```python
from build123d import *

# Parameters (mm, degrees)
F0_W     = 41.5
F0_H     = 36.8
F1_DEPTH = 20
F2_W     = 55
F2_H     = 2.5
F3_DEPTH = 20
F4_R     = 3
F5_DEPTH = 5
F6_R     = 2.25
F7_DEPTH = 25
F8_R     = 2


with BuildPart() as f1:
    # F0 (on Front) → F1 (new body)
    with BuildSketch(Plane.XZ):
        Rectangle(F0_W, F0_H)
    extrude(amount=F1_DEPTH)

    # F2 (on face) → F3 (join)
    with BuildSketch(Plane.XZ.offset(20)):
        with Locations((0, -11.15)):
            Rectangle(F2_W, F2_H)
    extrude(amount=-F3_DEPTH)

    # F4 (on face) → F5 (join)
    with BuildSketch(Plane(origin=(0, 0, -18.4), x_dir=(1, 0, 0), z_dir=(0, 0, -1))):
        with Locations((-10.75, 10)):
            Circle(F4_R)
    extrude(amount=F5_DEPTH)

    # F6 (on face) → F7 (cut)
    with BuildSketch(Plane(origin=(0, 0, -12.4), x_dir=(1, 0, 0), z_dir=(0, 0, -1))):
        with Locations((-25.5, 15)):
            Circle(F6_R)
        with Locations((-25.5, 5)):
            Circle(F6_R)
        with Locations((25.5, 15)):
            Circle(F6_R)
        with Locations((25.5, 5)):
            Circle(F6_R)
    extrude(amount=-F7_DEPTH, mode=Mode.SUBTRACT)

    # F8
    f8_edges = [f1.edges().sort_by_distance(p)[0] for p in [
        (27.5, -20, -11.15),
        (27.5, 0, -11.15),
        (-27.5, -20, -11.15),
        (-27.5, 0, -11.15),
    ]]
    fillet(f8_edges, radius=F8_R)


solid = f1.part
```
Geometry check sheet. Reference: the model listing, model coordinates, mm. A direction names the side the tool comes from. Give positions to 0.01 mm unless a question says otherwise; leave off trailing zeros. Write each loop counter-clockwise with the first axis right and the second up, starting at its lowest first coordinate (ties: lowest second). Pieces come first, ordered by that corner, then holes. Notation, with made-up numbers: (4, 40.25) -> (57, 40.25) arc R12 cw to (57, 50.25) -> close; hole circle Ø9 at (-34.75, -10). An arc over 180 degrees is marked (long way). Use one line per item in the form item = value.
Item 1: Sectioned sample at A-A on x = -10.75. Enter the section's corners in (y, z).
Results list:
outline = (-20, -18.4) -> (-13, -18.4) -> (-13, -23.4) -> (-7, -23.4) -> (-7, -18.4) -> (0, -18.4) -> (0, 18.4) -> (-20, 18.4) -> close
Item 2: Depth check by flat-ended pin: pin 1 Ø6 at (x, y) = (-1, -16) entering from -Z; pin 2 Ø6.5 at (y, z) = (-10.5, -16.5) entering from +X; pin 3 Ø5 at (x, y) = (25.5, -15) entering from -Z; pin 4 Ø5 at (x, z) = (14.5, -16.5) entering from +Y. Enter the tip coordinate at first touch or a pass-through.
Results list:
pin_1 = -18.4
pin_2 = 20.75
pin_3 = -12.4
pin_4 = 0
Item 3: Access from +Z, -Z, +X, -X, +Y, -Y to the whole of each face (thin tool, end or side, straight path). Record for faces 1 (the flat face through (23, -10, -12.4)), 2 (the flat face through (-20.75, -10, -15)), 3 (the cylindrical face through (-23.25, -4.92, -11.17)).
Results list:
face_1 = -Z, +X, +Y, -Y
face_2 = -Z, -X, +Y, -Y
face_3 = +Z, -Z
Item 4: Scan lines: line 1 (Y direction, x = -25.5, z = -10.55); line 2 (Z direction, x = 3.5, y = -10.75); line 3 (X direction, y = -4, z = -5.5). Record each from-to range of solid material in increasing order.
Results list:
line_1 = -20 to -17.25, -12.75 to -7.25, -2.75 to 0
line_2 = -18.4 to 18.4
line_3 = -20.75 to 20.75
Item 5: Sectioned sample at B-B on y = -10. Enter the section's corners in (x, z).
Results list:
outline = (-27.5, -12.4) -> (-20.75, -12.4) -> (-20.75, -18.4) -> (-13.75, -18.4) -> (-13.75, -23.4) -> (-7.75, -23.4) -> (-7.75, -18.4) -> (20.75, -18.4) -> (20.75, -12.4) -> (27.5, -12.4) -> (27.5, -9.9) -> (20.75, -9.9) -> (20.75, 18.4) -> (-20.75, 18.4) -> (-20.75, -9.9) -> (-27.5, -9.9) -> close
Item 6: Sectioned sample at D-D on y = -5. Enter the section's corners in (x, z).
Results list:
outline = (-23.25, -12.4) -> (-20.75, -12.4) -> (-20.75, -18.4) -> (20.75, -18.4) -> (20.75, -12.4) -> (23.25, -12.4) -> (23.25, -9.9) -> (20.75, -9.9) -> (20.75, 18.4) -> (-20.75, 18.4) -> (-20.75, -9.9) -> (-23.25, -9.9) -> close
Item 7: Sectioned sample at C-C on z = -4. Enter the section's corners in (x, y), plus the area to 3 significant figures.
Results list:
outline = (-20.75, -20) -> (20.75, -20) -> (20.75, 0) -> (-20.75, 0) -> close
area = 830 mm2
Item 8: Mould release check, pull along Y, two halves, no side actions. Record for faces 4 (the cylindrical face through (-26.93, -19.4, -11.13)), 5 (the cylindrical face through (23.25, -5.08, -11.17)), 6 (the flat face through (20.75, -10, -15)): released by +Y, released by -Y, zero draft, split by the parting line, or undercut.
Results list:
face_4 = released by -Y
face_5 = undercut
face_6 = zero draft
